Here's the drawing with two shaded views (mm, measured from the low corner). I have some questions. Round coordinates to 2 decimals unless told otherwise and drop trailing zeros. Write each loop counter-clockwise with the first axis right and the second up, starting at its lowest first coordinate (ties: lowest second). Pieces come first, ordered by that corner, then holes. Notation, with made-up numbers: (8.5, -3.75) -> (56.5, -3.75) arc R19 cw to (56.5, 7.25) -> close; hole circle Ø11 at (-8.75, 14.5). An arc over 180 degrees is marked (long way). Use CSV: the item, a comma, the result in double quotes.
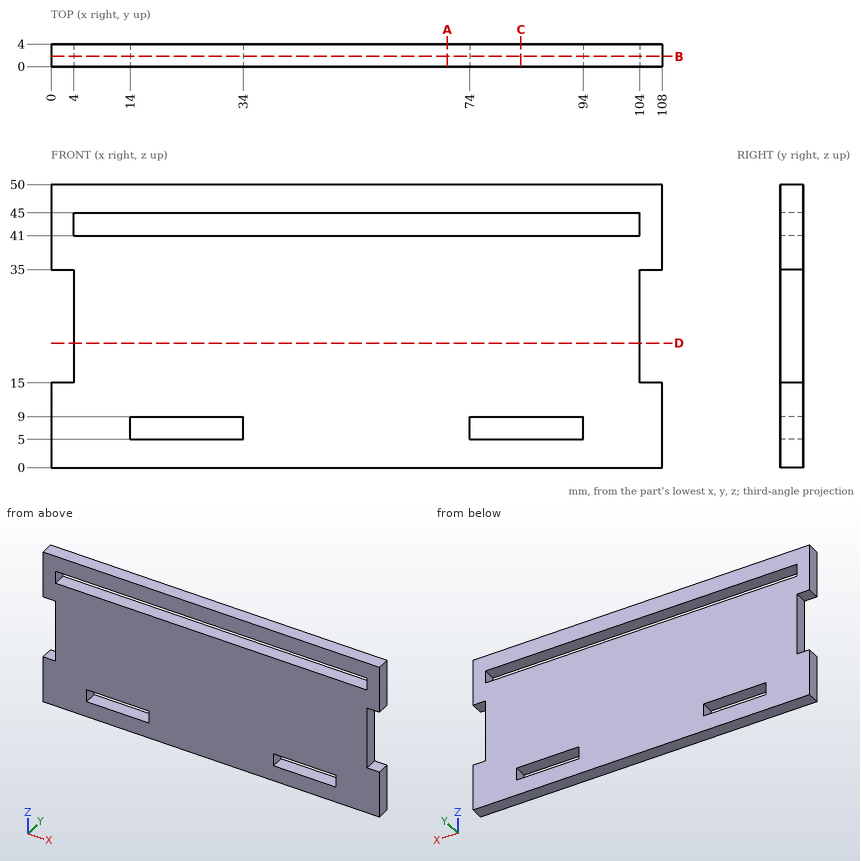
Q1. Suppose I cut it at C-C (x = 83). Write out the boundary of the cut face in (y, z).
Resolved:
outline,"(0, 0) -> (4, 0) -> (4, 5) -> (0, 5) -> close; (0, 9) -> (4, 9) -> (4, 41) -> (0, 41) -> close; (0, 45) -> (4, 45) -> (4, 50) -> (0, 50) -> close"
Q2. Suppose I cut it at B-B (y = 1.8). Write out the boundary of the cut face in (x, z).
Resolved:
outline,"(0, 0) -> (108, 0) -> (108, 15) -> (104, 15) -> (104, 35) -> (108, 35) -> (108, 50) -> (0, 50) -> (0, 35) -> (4, 35) -> (4, 15) -> (0, 15) -> close; hole (4, 41) -> (104, 41) -> (104, 45) -> (4, 45) -> close; hole (14, 5) -> (34, 5) -> (34, 9) -> (14, 9) -> close; hole (74, 5) -> (94, 5) -> (94, 9) -> (74, 9) -> close"
Q3. Suppose I cut it at D-D (z = 22). Write out the boundary of the cut face in (x, y), and give its area (3 significant figures).
Resolved:
outline,"(4, 0) -> (104, 0) -> (104, 4) -> (4, 4) -> close"
area,"400 mm^2"
Q4. Will these pins go through, and if not, where does the flat tip stop? P1, Ø2, axis at y = 2.5, z = 27.5, coming from the -X side; P2, Ø2, axis at y = 2.5, z = 29.5, coming from the +X side.
Resolved:
P1,"stops at x = 4"
P2,"stops at x = 104"
Q5. Please list where these lines run through material, in increasing order: probe 1 along X at (y, z) = (1.55, 8); probe 2 along Z at (x, y) = (92.5, 0.75); probe 3 along Z at (x, y) = (68.5, 1.15).
Resolved:
probe 1,"x = 0 to 14, 34 to 74, 94 to 108"
probe 2,"z = 0 to 5, 9 to 41, 45 to 50"
probe 3,"z = 0 to 41, 45 to 50"
Q6. Suppose I cut it at A-A (x = 70). Write out the boundary of the cut face in (y, z).
Resolved:
outline,"(0, 0) -> (4, 0) -> (4, 41) -> (0, 41) -> close; (0, 45) -> (4, 45) -> (4, 50) -> (0, 50) -> close"
